from build123d import *

# Parameters (mm, degrees)
F0_W     = 12.2949928045
F0_H     = 111.9073554873
F1_DEPTH = 25.4
F2_DEPTH = 50.8
F3_R     = 9.6329205763
F3_R_2   = 10.3143996585
F3_R_3   = 9.7245159321
F3_R_4   = 10.9939674149
F3_R_5   = 9.8001864777
F4_DEPTH = 50.8


with BuildPart() as f1:
    # F0 (on Top) → F1 (new body)
    with BuildSketch(Plane.XY):
        with Locations((6.1474964023, 55.9536777437)):
            Rectangle(F0_W, F0_H)
        Polygon((12.2949928045, 0), (0, 0), (-124.18808043, 0), (-97.1772074699, -43.5698479414), (-11.5329865366, -85.7331603765), (74.1112306714, -85.7331603765), (114.9569302797, -56.087076664), (138.0150020123, 0), align=None)
        Polygon((0, 213.3628129959), (0, 111.9073554873), (12.2949928045, 111.9073554873), (97.8280827403, 111.9073554873), align=None)
    extrude(amount=F1_DEPTH)

    # F0 (on Top) → F2 (join)
    with BuildSketch(Plane.XY):
        with Locations((6.1474964023, 55.9536777437)):
            Rectangle(F0_W, F0_H)
        Polygon((12.2949928045, 0), (0, 0), (-124.18808043, 0), (-97.1772074699, -43.5698479414), (-11.5329865366, -85.7331603765), (74.1112306714, -85.7331603765), (114.9569302797, -56.087076664), (138.0150020123, 0), align=None)
        Polygon((0, 213.3628129959), (0, 111.9073554873), (12.2949928045, 111.9073554873), (97.8280827403, 111.9073554873), align=None)
    extrude(amount=F2_DEPTH)

    # F3 (on face) → F4 (cut)
    with BuildSketch(Plane.XY.offset(50.8)):
        with Locations((24.2112372071, -16.715940088)):
            Circle(F3_R)
        with Locations((54.1940517724, -15.5627541244)):
            Circle(F3_R_2)
        with Locations((81.1017081141, -14.7939696908)):
            Circle(F3_R_3)
        with Locations((-69.5811584592, -17.4847338349)):
            Circle(F3_R_4)
        with Locations((-32.2948358953, -16.3315478712)):
            Circle(F3_R_5)
    extrude(amount=-F4_DEPTH, mode=Mode.SUBTRACT)


solid = f1.part
Verification items for the finished model (mm, model axes). A direction names the side the tool comes from. Give positions to 0.01 mm unless a question says otherwise; leave off trailing zeros. Write each loop counter-clockwise with the first axis right and the second up, starting at its lowest first coordinate (ties: lowest second). Pieces come first, ordered by that corner, then holes.
(1) Access from +Z, -Z, +X, -X, +Y, -Y to the whole of each face (thin tool, end or side, straight path). Record for faces 4 (the face through (14.588, -16.292, 25.756)), 5 (the face through (12.295, 55, 25)), 6 (the face through (-61, 0, 25)).
(2) Material ranges on line 1 (Y direction, x = 45, z = 4.5); line 2 (X direction, y = -9, z = 23.5) (3 decimals); line 3 (Y direction, x = 83, z = 46.5), recorded low to high.
(3) Gauge pin test, flat ends, axial feed: pin 1 (4 mm diameter, centred on x = 84, z = 6, fed in from +Y); pin 2 (2 mm diameter, centred on y = 147, z = 16, fed in from -X); pin 3 (6 mm diameter, centred on x = 59, z = 39, fed in from +Y). Record the tip position at first contact, or that the pin passes through.
(4) Cross-section at A-A (x = -27). Enter the section's corners in (y, z).
(5) Cross-section at C-C (x = 85.5). Enter the section's corners in (y, z).
(6) Cross-section at D-D (y = 173). Enter the section's corners in (x, z).
(7) Mould release check, pull along Y, two halves, no side actions. Record for faces 1 (the face through (-54.95, -64.36, 25.04)), 2 (the face through (90.377, -11.873, 25.756)), 3 (the face through (5, 33, 0)): +Y half, -Y half, draft (parallel to the pull), parting line (faces both ways), or undercut.
(8) Cross-section at B-B (z = 40). Enter the section's corners in (x, y) (3 decimals).
Worked out:
1. face 4: +Z, -Z
1. face 5: +Z, -Z, +X
1. face 6: +Z, -Z, -X, +Y
2. line 1: y = -85.73 to -20.24, -10.89 to 0, 111.91 to 166.69
2. line 2: x = -118.609 to -76.572, -62.59 to -38.798, -25.792 to 18.444, 29.978 to 46.237, 62.151 to 73.292, 88.912 to 134.315
2. line 3: y = -79.28 to -24.33, -5.26 to 0, 111.91 to 127.29
3. pin 1: stops at y = 128.32
3. pin 2: stops at x = 0
3. pin 3: stops at y = 155.29
4. outline: (-78.12, 0) - (-24.58, 0) - (-24.58, 50.8) - (-78.12, 50.8) - close; (-8.08, 0) - (0, 0) - (0, 50.8) - (-8.08, 50.8) - close
5. outline: (-77.47, 0) - (-23.47, 0) - (-23.47, 50.8) - (-77.47, 50.8) - close; (-6.12, 0) - (0, 0) - (0, 50.8) - (-6.12, 50.8) - close; (111.91, 0) - (124.69, 0) - (124.69, 50.8) - (111.91, 50.8) - close
6. outline: (0, 0) - (38.92, 0) - (38.92, 50.8) - (0, 50.8) - close
7. face 1: -Y half
7. face 2: undercut
7. face 3: draft
8. outline: (-124.188, 0) - (-97.177, -43.57) - (-11.533, -85.733) - (74.111, -85.733) - (114.957, -56.087) - (138.015, 0) - (12.295, 0) - (12.295, 111.907) - (97.828, 111.907) - (0, 213.363) - (0, 0) - close; hole circle Ø21.988 at (-69.581, -17.485); hole circle Ø19.6 at (-32.295, -16.332); hole circle Ø19.266 at (24.211, -16.716); hole circle Ø20.629 at (54.194, -15.563); hole circle Ø19.449 at (81.102, -14.794)
